The model under review builds one solid part; all positions refer to its coordinate system, in mm. A direction names the side the tool comes from. Coordinates: 2 decimals unless noted, no trailing zeros. Write each loop counter-clockwise with the first axis right and the second up, starting at its lowest first coordinate (ties: lowest second). Pieces come first, ordered by that corner, then holes.
1) Add section A-A, the plane y = -7. State the section outline as (x, z) points.
2) Add section D-D, the plane y = 13.5. State the section outline as (x, z) points.
3) Machinability: for faces 1 (the flat face through (-11.4, 19, 3)), 2 (the flat face through (7.4, 20, 2)), 3 (the flat face through (17.454, -4, 4)), 4 (the flat face through (7.4, -20, 2)), 5 (the flat face through (-9, 19, 1)), which of the approach directions +Z, -Z, +X, -X, +Y, -Y give a long, thin tool a straight path to every point of the face, cutting with its end or side? Answer none if there is none.
4) For line 1 (Y direction, x = -0.5, z = 2.4); line 2 (Y direction, x = 10, z = 2.5), list the stretches that pass through material, from the lowest coordinate up.
5) Add section C-C, the plane x = -16. State the section outline as (y, z) points, then the cut area to 3 significant figures.
6) For P1, Ø0.8, axis at x = -8, y = -19, coming from the -Z side; P2, Ø1.5, axis at y = -15, z = 3, coming from the -X side; P3, Ø2.5, axis at y = 19, z = 2.5, coming from the -X side, all flat-tipped, find the tip position at first contact; note any pin that passes through.
7) Add section B-B, the plane x = 5. State the section outline as (y, z) points, then the cut area to 3 significant figures.
8) Mouldability with a two-part tool opening along Z and no side actions: class faces 6 (the flat face through (14.468, 14.374, 0.406)), 7 (the flat face through (15.95, 1, 4)), 8 (the flat face through (-17, 6.45, 3)) as released by +Z, released by -Z, zero draft, split by the parting line, or undercut.
from build123d import *

# Parameters (mm, degrees)
PAD_DEPTH               = 5
POCKET_DEPTH            = 4.5
POCKET001_DEPTH         = 3
SKETCH005_W             = 2.9792998166
SKETCH005_H             = 2.1103373701
PAD001_DEPTH            = 0.7
POCKET002_DEPTH         = 2.5
POCKET003_DEPTH         = 3
PAD002_DEPTH            = 4
PAD002_MIRRORED_2_DEPTH = 4
SKETCH014_R             = 0.4
POCKET004_DEPTH         = 140.0632958807
SKETCH003_W             = 4.4
SKETCH003_H             = 6.4
POCKET005_DEPTH         = 0.501
CHAMFER_SIZE            = 0.8
CHAMFER001_SIZE         = 0.4


with BuildPart() as part:
    # Sketch001 → Pad (new body)
    with BuildSketch(Plane.XY):
        Polygon((18.05, 11.35), (11.35, 18.05), (-11.35, 18.05), (-18.05, 11.35), (-18.05, -11.35), (-11.35, -18.05), (11.35, -18.05), (18.05, -11.35), align=None)
    extrude(amount=PAD_DEPTH)

    # Sketch (on Face10 of Pad) → Pocket (cut)
    with BuildSketch(Plane.XY.offset(5)):
        Polygon((-15.2, 10.1176776962), (-15.2, -10.1176776962), (-10.1, -15.2), (10.1, -15.2), (15.2, -10.1176776962), (15.2, 10.1176776962), (10.1, 15.2), (-10.1, 15.2), align=None)
    extrude(amount=-POCKET_DEPTH, mode=Mode.SUBTRACT)

    # Sketch004 (on Face19 of Pocket) → Pocket001 (cut)
    with BuildSketch(Plane.XY.offset(1.25)):
        Polygon((15.2, 3.4), (15.2, 7.2), (16.7, 7.2), (16.7, 6.45), (18.2, 6.45), (18.2, 4.15), (16.7, 4.15), (16.7, 3.4), align=None)
        Polygon((-15.2, 3.4), (-15.2, 7.2), (-16.7, 7.2), (-16.7, 6.45), (-18.2, 6.45), (-18.2, 4.15), (-16.7, 4.15), (-16.7, 3.4), align=None)
    extrude(amount=POCKET001_DEPTH, mode=Mode.SUBTRACT)

    # Sketch005 (on Face31 of Pocket001) → Pad001 (join)
    with BuildSketch(Plane.XY.offset(0.5)):
        Polygon((-10.1, 15.2), (-10.1, 12.2207001834), (-12.2103373701, 10.1176776962), (-15.2, 10.1176776962), align=None)
        Polygon((12.2103373701, 10.1176776962), (15.2, 10.1176776962), (10.1, 15.2), (10.1, 12.2207001834), align=None)
        with Locations((4.6103500917, -14.1448313149)):
            Rectangle(SKETCH005_W, SKETCH005_H)
    extrude(amount=PAD001_DEPTH)

    # Sketch006 → Pocket002 (cut, symmetric)
    with BuildSketch(Plane.XZ):
        Polygon((-18.2, 5), (-18.2, 2), (-16.7, 3), (-17.2, 3.5), (-17.2, 5), align=None)
    extrude(amount=POCKET002_DEPTH, both=True, mode=Mode.SUBTRACT)

    # Sketch007 → Pocket003 (cut)
    with BuildSketch(Plane.XY.offset(5)):
        with BuildLine():
            ThreePointArc((15.95, 0.5), (16.7, -0.25), (17.45, 0.5))
            Line((17.45, 0.5), (17.45, 2.25))
            ThreePointArc((17.45, 2.25), (16.7000041345, 3.0000082691), (15.95, 2.2500082691))
            Line((15.95, 0.5), (15.95, 2.2500082691))
        make_face()
        with BuildLine():
            ThreePointArc((15.9543057832, -5.2499990728), (16.7043057832, -5.9999990728), (17.4543057832, -5.2499990728))
            Line((17.4543057832, -5.2499990728), (17.4543057832, -3.4999990728))
            ThreePointArc((17.4543057832, -3.4999990728), (16.7043053195, -2.75), (15.9543057832, -3.5))
            Line((15.9543057832, -5.2499990728), (15.9543057832, -3.5))
        make_face()
    extrude(amount=-POCKET003_DEPTH, mode=Mode.SUBTRACT)

    # Sketch008 → Pad002 (join)
    with BuildSketch(Plane.YZ.offset(7.4)):
        Polygon((-18, 1), (-18, 5), (-20.8, 3), (-20.8, 1), align=None)
    pad002 = extrude(amount=PAD002_DEPTH)

    # Sketch008 Mirrored 2 → Pad002 Mirrored 2 (add)
    with BuildSketch(Plane(origin=(7.4, 0, 0), x_dir=(0, -1, 0), z_dir=(-1, 0, 0))):
        Polygon((-18, 1), (-18, 5), (-20.8, 3), (-20.8, 1), align=None)
    pad002_mirrored_2 = extrude(amount=-PAD002_MIRRORED_2_DEPTH)

    # Mirrored001: Pad002, Pad002 Mirrored 2 across YZ
    add(pad002.mirror(Plane.YZ))
    add(pad002_mirrored_2.mirror(Plane.YZ))

    # Sketch014 (on Face59 of MultiTransform) → Pocket004 (cut, through all)
    with BuildSketch(Plane.YZ.offset(11.4)):
        with Locations((-19.4, 2.3)):
            Circle(SKETCH014_R)
    pocket004 = extrude(amount=-POCKET004_DEPTH, mode=Mode.SUBTRACT)

    # Mirrored002: Pocket004 across Sketch014 V_Axis
    add(pocket004.mirror(Plane(origin=(11.4, 0, 0), x_dir=(1, 0, 0), z_dir=(0, 1, 0))), mode=Mode.SUBTRACT)

    # Sketch003 (on Face67 of Mirrored002) → Pocket005 (cut, through all)
    with BuildSketch(Plane.XY.offset(0.5)):
        Rectangle(SKETCH003_W, SKETCH003_H)
    extrude(amount=-POCKET005_DEPTH, mode=Mode.SUBTRACT)

    # Chamfer
    chamfer_edges = [part.edges().sort_by_distance(p)[0] for p in [
        (-14.7, -14.7, 0),
        (-18.05, 0, 0),
        (0, 18.05, 0),
        (-14.7, 14.7, 0),
        (14.7, 14.7, 0),
        (18.05, 0, 0),
        (14.7, -14.7, 0),
        (0, -18.05, 0),
    ]]
    chamfer(chamfer_edges, length=CHAMFER_SIZE)

    # Chamfer001
    chamfer001_edges = [part.edges().sort_by_distance(p)[0] for p in [
        (7.4, 18.05, 2.982143),
        (-7.4, 18.05, 2.982143),
        (-7.4, -18.05, 2.982143),
        (7.4, -18.05, 2.982143),
    ]]
    chamfer(chamfer001_edges, length=CHAMFER001_SIZE)


solid = part.part
Geometry results:
1. outline: (-18.05, 0.8) - (-17.25, 0) - (17.25, 0) - (18.05, 0.8) - (18.05, 5) - (15.2, 5) - (15.2, 0.5) - (-15.2, 0.5) - (-15.2, 5) - (-18.05, 5) - close
2. outline: (-15.9, 0.8) - (-14.77, 0) - (14.77, 0) - (15.9, 0.8) - (15.9, 5) - (11.81, 5) - (11.81, 1.2) - (10.1, 1.2) - (10.1, 0.5) - (-10.1, 0.5) - (-10.1, 1.2) - (-11.81, 1.2) - (-11.81, 5) - (-15.9, 5) - close
3. face 1: +Z, -Z, -X, +Y
3. face 2: +Z, -Z, +Y
3. face 3: +Z
3. face 4: +Z, -Z, -Y
3. face 5: -Z, +X, -X, +Y
4. line 1: y = -18.05 to -15.2, 15.2 to 18.05
4. line 2: y = -20.8 to -19.75, -19.05 to -15.2, 15.2 to 19.05, 19.75 to 20.8
5. outline: (-13.4, 0.8) - (-12.27, 0) - (12.27, 0) - (13.4, 0.8) - (13.4, 5) - (-13.4, 5) - close; hole (3.4, 1.25) - (7.2, 1.25) - (7.2, 4.25) - (3.4, 4.25) - close
5. area: 122 mm2
6. P1: stops at z = 1
6. P2: stops at x = -15.15
6. P3: stops at x = -11.65
7. outline: (-18.05, 0.8) - (-17.25, 0) - (17.25, 0) - (18.05, 0.8) - (18.05, 5) - (15.2, 5) - (15.2, 0.5) - (-13.09, 0.5) - (-13.09, 1.2) - (-15.2, 1.2) - (-15.2, 5) - (-18.05, 5) - close
7. area: 44.5 mm2
8. face 6: released by -Z
8. face 7: zero draft
8. face 8: undercut
